Could you check a few things on this model? Use its own coordinates, in mm. Face numbers are marked on the shaded views. A direction names the side the tool comes from. Give positions to 0.01 mm unless a question says otherwise; leave off trailing zeros. Loops run counter-clockwise (first coordinate to the right, second up) from the corner with the lowest first, then second, coordinate; pieces in that order, holes last. Notation, with made-up numbers: M 89.5,-7 L 126.5,-7 A19 ccw 126.5,7 Z; hole C 48,31.25 d3. An arc over 180 degrees is marked long. Answer in a Markdown table with one row per item. Add a question column.
```python
from build123d import *

# Parameters (mm, degrees)
F1_DEPTH    = 50
F2_R        = 5
F3_T1_DEPTH = 61.0584684806
F3_T3_DEPTH = 59.847165152
F3_T5_DEPTH = 60
F4_R        = 5
F5_W        = 35.3398231359
F5_H        = 20
F5_W_2      = 28.4329991749
F6_DEPTH    = 102.5
F8_DEPTH    = 25


# Not quite as in the source:
# - a fillet or chamfer that OpenCascade refuses, or shapes differently, is made with other operations: its cross-section is extruded or revolved along the edge and cut away or added


with BuildPart() as f1:
    # F0 (on Front) → F1 (new body)
    with BuildSketch(Plane.XZ):
        with BuildLine():
            ThreePointArc((31.8191999969, 11.4080709653), (17.9368952367, 8.7096242744), (15.2384485458, 22.5919290347))
            Line((15.2384485458, 22.5919290347), (67.0269365518, 99.3715199707))
            Line((67.0269365518, 99.3715199707), (61.2236735439, 103.285870295))
            Line((61.2236735439, 103.285870295), (2.7757529523, 16.6332645351))
            ThreePointArc((2.7757529523, 16.6332645351), (-7.6399843, 21.3751609063), (-6.7842885115, 32.7874765531))
            Line((-6.7842885115, 32.7874765531), (-9.6689994545, 34.7836766193))
            ThreePointArc((-9.6689994545, 34.7836766193), (-11.3082346995, 20.8471863165), (0.3142037122, 12.9838677097))
            Line((0.3142037122, 12.9838677097), (-5.8783996854, 3.8029556189))
            Line((-5.8783996854, 3.8029556189), (0, 0))
            Line((0, 0), (32.5678846096, 0))
            Line((32.5678846096, 0), (60.1479586957, 40.8891413488))
            Line((60.1479586957, 40.8891413488), (87.7280327819, 0))
            Line((87.7280327819, 0), (96.1715584214, 0))
            Line((96.1715584214, 0), (64.3697215155, 47.1481621237))
            Line((64.3697215155, 47.1481621237), (58.5664585076, 51.062512448))
            Line((58.5664585076, 51.062512448), (31.8191999969, 11.4080709653))
        make_face()
    extrude(amount=F1_DEPTH)

    # F2
    f2_edges = [f1.edges().sort_by_distance(p)[0] for p in [
        (58.566459, -25, 51.062512),
        (60.147959, -25, 40.889141),
        (32.567885, -25, 0),
        (87.728033, -25, 0),
        (0, -25, 0),
        (-5.8784, -25, 3.802956),
    ]]
    fillet(f2_edges, radius=F2_R)

    # F3: fillet of radius 2 on 4 edges, made by hand

    # F3_s2 → F3_t1 (cut)
    with BuildSketch(Plane.XZ.offset(-5.5292342403)):
        with BuildLine():
            ThreePointArc((-10.8840299501, 32.9356263223), (-9.5901444427, 33.9234656813), (-7.9904107365, 33.6221048098))
            Line((-7.9904107365, 33.6221048098), (-9.6689994545, 34.7836766193))
            ThreePointArc((-9.6689994545, 34.7836766193), (-10.3144239688, 33.8845755298), (-10.8840299501, 32.9356263223))
        make_face()
    extrude(amount=F3_T1_DEPTH, mode=Mode.SUBTRACT)

    # F3_s4 → F3_t3 (cut)
    with BuildSketch(Plane.XZ.offset(-4.923582576)):
        with BuildLine():
            ThreePointArc((-8.4037793712, 33.9081530525), (-7.5948464442, 32.7208873787), (-7.790553617, 31.2976266988))
            ThreePointArc((-7.790553617, 31.2976266988), (-7.3209703374, 32.065211267), (-6.7842885115, 32.7874765531))
            Line((-6.7842885115, 32.7874765531), (-8.4037793712, 33.9081530525))
        make_face()
    extrude(amount=F3_T3_DEPTH, mode=Mode.SUBTRACT)

    # F3_s6 → F3_t5 (cut)
    with BuildSketch(Plane.XZ.offset(-5)):
        with BuildLine():
            ThreePointArc((60.105287737, 101.6277951499), (61.3817448913, 102.4726637098), (62.881748689, 102.1674844881))
            Line((62.881748689, 102.1674844881), (61.2236735439, 103.285870295))
            Line((61.2236735439, 103.285870295), (60.105287737, 101.6277951499))
        make_face()
        with BuildLine():
            ThreePointArc((65.3688614067, 100.4899057776), (66.2137299667, 99.2134486233), (65.9085507449, 97.7134448256))
            Line((65.9085507449, 97.7134448256), (67.0269365518, 99.3715199707))
            Line((67.0269365518, 99.3715199707), (65.3688614067, 100.4899057776))
        make_face()
    extrude(amount=F3_T5_DEPTH, mode=Mode.SUBTRACT)

    # F4
    f4_edges = [f1.edges().sort_by_distance(p)[0] for p in [
        (2.775753, -25, 16.633265),
        (0.314204, -25, 12.983868),
    ]]
    fillet(f4_edges, radius=F4_R)

    # F5 (on face) → F6 (cut)
    with BuildSketch(Plane(origin=(0, 0, 0), x_dir=(1, 0, 0), z_dir=(0, 0, -1))):
        with Locations((-16.1935732915, 25)):
            Rectangle(F5_W, F5_H)
        with Locations((15.6928378639, 25)):
            Rectangle(F5_W_2, F5_H)
        with BuildLine():
            Line((29.9093374513, 15), (38.8109274209, 15))
            ThreePointArc((38.8109274209, 15), (48.8109274209, 25), (38.8109274209, 35))
            Line((38.8109274209, 35), (29.9093374513, 35))
            Line((29.9093374513, 35), (29.9093374513, 15))
        make_face()
    extrude(amount=-F6_DEPTH, mode=Mode.SUBTRACT)

    # F7 (on face) → F8 (cut)
    with BuildSketch(Plane(origin=(66.0990291526, 0, 44.5843581184), x_dir=(0, 1, 0), z_dir=(0.8290375726, 0, 0.5591929035))):
        with BuildLine():
            Line((-15, -53.778452985), (-15, -17.8613532335))
            ThreePointArc((-15, -17.8613532335), (-25, -7.8613532335), (-35, -17.8613532335))
            Line((-35, -17.8613532335), (-35, -53.778452985))
            Line((-35, -53.778452985), (-15, -53.778452985))
        make_face()
    extrude(amount=-F8_DEPTH, mode=Mode.SUBTRACT)


solid = f1.part
```
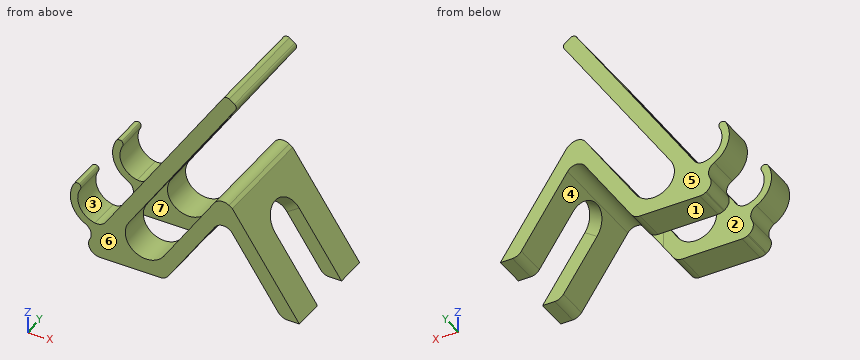
Item 1: Suppose I cut it at A-A (x = 19). List the corners of the cut face in (y, z) for me.
Item 2: I need wall thicknesses on L1, parallel to X at y = -41.5, z = 16; L2, parallel to X at y = -1.5, z = 35.5; L3, parallel to X at y = -6, z = 26.5. Which ranges of each line are inside material? Lowest first, please.
Item 3: Suppose I cut it at D-D (z = 24). Give the number of separate pieces and of enclosed holes in the cut face, then the cut area to 3 significant figures.
Item 4: Suppose I cut it at C-C (z = 43). List the corners of the cut face in (x, y) for me.
Item 5: For P1, Ø2, axis at y = -31.5, z = 40.5, coming from the -X side; P2, Ø10, axis at y = -6, z = 48.5, coming from the -X side; P3, Ø12, axis at x = 44, y = -6.5, coming from the -Z side, each with a flat end and sliding along its axis, tell me the tip position at first contact or that it passes through.
Item 6: For the marked faces 1, 2 and 3, which set-ups out of +Z, -Z, +X, -X, +Y, -Y let a thin tool reach every point of the face, with its end or its side?
Item 7: If we mould it in two halves opening along Y, with no side actions, what happens to the marked faces 4, 5, 6 and 7? For each: +Y half, -Y half, draft (parallel to the pull), parting line (faces both ways), or undercut.
Item 8: Suppose I cut it at B-B (y = -25). List the corners of the cut face in (x, z) for me.
Values found:
| question | item | result |
|---|---|---|
| 1 | outline | M -50,0 L -35,0 L -35,8.08 L -50,8.08 Z; M -50,28.17 L -35,28.17 L -35,40.69 L -50,40.69 Z; M -15,0 L 0,0 L 0,8.08 L -15,8.08 Z; M -15,28.17 L 0,28.17 L 0,40.69 L -15,40.69 Z |
| 2 | L1 | -7.56 to 13.58, 34.92 to 43.36, 76.94 to 85.38 |
| 2 | L2 | 15.5 to 23.95, 48.07 to 56.63, 63.67 to 72.23 |
| 2 | L3 | -12.53 to -9.03, 9.43 to 17.87, 42 to 50.44, 69.85 to 78.3 |
| 3 | separate pieces | 8 |
| 3 | enclosed holes | 0 |
| 3 | area | 909 mm² |
| 4 | outline | M 20.56,-50 L 29,-50 L 29,-35 L 20.56,-35 Z; M 20.56,-15 L 29,-15 L 29,0 L 20.56,0 Z; M 53.13,-50 L 67.17,-50 L 67.17,0 L 53.13,0 Z |
| 5 | P1 | x = 50.77 |
| 5 | P2 | x = 20.9 |
| 5 | P3 | z = 8.05 |
| 6 | face 1 | -Z, +X, -X, +Y, -Y |
| 6 | face 2 | +Z, -Z, -X |
| 6 | face 3 | +Y, -Y |
| 7 | face 4 | draft |
| 7 | face 5 | +Y half |
| 7 | face 6 | -Y half |
| 7 | face 7 | undercut |
| 8 | outline | M 48.81,24.08 L 56,34.74 A5 cw 64.29,34.74 L 64.69,34.15 L 70.5,38.07 L 64.37,47.15 L 62.71,48.27 A5 ccw 55.77,46.92 L 48.81,36.6 Z; M 48.81,72.37 L 65.91,97.71 A2 ccw 65.37,100.49 L 62.88,102.17 A2 ccw 60.11,101.63 L 48.81,84.88 Z |
